Verification items for the finished model (mm, model axes). Face numbers are marked on the shaded views. Give positions to 0.01 mm unless a question says otherwise; leave off trailing zeros. Order: outer loops, then holes, each group sorted by start corner. A loop starts at its lowest first (then second) coordinate and runs counter-clockwise, first axis right, second up. Notation, with made-up numbers: (43, 72.5) - (51, 72.5) arc R24 ccw to (51, 106.5) - close; hole circle Ø5 at (-12, -5.75). An arc over 180 degrees is marked (long way). Answer as a JSON object with one key per item and string values. Group by question number.
(1) Section check B-B (x = -9.5). Record the boundary of the cut face in (y, z), then the cut area to 3 significant figures.
(2) Mould release check, pull along Z, two halves, no side actions. Record for the marked faces 1 and 2: +Z half, -Z half, draft (parallel to the pull), parting line (faces both ways), or undercut.
(3) Thickness scan on line 1 (X direction, y = 0.25, z = -8); line 2 (Z direction, x = -30, y = 1.65); line 3 (X direction, y = 2.35, z = -24). Record the ranges inside material, lowest first.
(4) Depth check by flat-ended pin: pin 1 Ø3.5 at (x, z) = (31.46, 22.98) entering from +Y; pin 2 Ø1.5 at (y, z) = (1, -19) entering from +X; pin 3 Ø1.7 at (y, z) = (1.5, -22) entering from +X; pin 4 Ø0.6 at (x, y) = (-1, 1) entering from +Z. Enter the tip coordinate at first touch or a pass-through.
(5) Section check A-A (z = 6.5). Record the boundary of the cut face in (x, y).
(6) Section check D-D (y = 3.45). Count the separate pieces of the cut face and the enclosed holes in it, then the cut area to 3 significant figures.
(7) Section check C-C (x = 31). Record the boundary of the cut face in (y, z), then the cut area to 3 significant figures.
```python
from build123d import *

# Parameters (mm, degrees)
SKETCH1_R           = 1.6
BOSS_EXTRUDE1_DEPTH = 4.1
CUT_EXTRUDE1_DEPTH  = 2
FILLET2_R           = 30
CUT_EXTRUDE4_DEPTH  = 3.1
SKETCH7_W           = 35
SKETCH7_H           = 20
CUT_EXTRUDE5_DEPTH  = 3.1


with BuildPart() as part:
    # Sketch1 → Boss-Extrude1 (new body)
    with BuildSketch(Plane(origin=(0, 0, 0), x_dir=(1, 0, 0), z_dir=(0, 1, 0))):
        Polygon((-12.5, 35), (12.5, 35), (23.684823703, 36.412745764), (36.412745764, 23.684823703), (35, 12.5), (35, -12.5), (36.412745764, -23.684823703), (23.684823703, -36.412745764), (12.5, -35), (-12.5, -35), (-23.684823703, -36.412745764), (-36.412745764, -23.684823703), (-35, -12.5), (-35, 12.5), (-36.412745764, 23.684823703), (-23.684823703, 36.412745764), align=None)
        with Locations((22.977716922, 31.462998296)):
            Circle(SKETCH1_R, mode=Mode.SUBTRACT)
        with Locations((31.462998296, 22.977716922)):
            Circle(SKETCH1_R, mode=Mode.SUBTRACT)
        with Locations((31.462998296, -22.977716922)):
            Circle(SKETCH1_R, mode=Mode.SUBTRACT)
        with Locations((22.977716922, -31.462998296)):
            Circle(SKETCH1_R, mode=Mode.SUBTRACT)
        with Locations((-22.977716922, -31.462998296)):
            Circle(SKETCH1_R, mode=Mode.SUBTRACT)
        with Locations((-31.462998296, -22.977716922)):
            Circle(SKETCH1_R, mode=Mode.SUBTRACT)
        with Locations((-31.462998296, 22.977716922)):
            Circle(SKETCH1_R, mode=Mode.SUBTRACT)
        with Locations((-22.977716922, 31.462998296)):
            Circle(SKETCH1_R, mode=Mode.SUBTRACT)
    extrude(amount=BOSS_EXTRUDE1_DEPTH)

    # Sketch2 → Cut-Extrude1 (cut)
    with BuildSketch(Plane(origin=(0, 4.1, 0), x_dir=(1, 0, 0), z_dir=(0, 1, 0))):
        Polygon((0, 0), (0, 29), (-4.760594582, 29), (-18.369647406, 29), (-29, 18.369647406), (-29, 0), align=None)
        Polygon((18.369647406, 29), (0, 29), (0, 0), (-29, 0), (-29, -18.369647406), (-18.369647406, -29), (18.369647406, -29), (29, -18.369647406), (29, 18.369647406), align=None)
    extrude(amount=-CUT_EXTRUDE1_DEPTH, mode=Mode.SUBTRACT)

    # Fillet2
    fillet2_edges = [part.edges().sort_by_distance(p)[0] for p in [
        (-12.5, 2.05, -35),
        (12.5, 2.05, -35),
        (35, 2.05, -12.5),
        (35, 2.05, 12.5),
        (12.5, 2.05, 35),
        (-12.5, 2.05, 35),
        (-35, 2.05, 12.5),
        (-35, 2.05, -12.5),
    ]]
    fillet(fillet2_edges, radius=FILLET2_R)

    # Sketch6 → Cut-Extrude4 (cut, through all)
    with BuildSketch(Plane(origin=(0, 2.1, 0), x_dir=(1, 0, 0), z_dir=(0, 1, 0))):
        with BuildLine():
            Line((-1.5, 19.7), (-1.5, 18.3))
            ThreePointArc((-1.5, 18.3), (-1.734314575, 17.734314575), (-2.3, 17.5))
            Line((-2.3, 17.5), (-6.7, 17.5))
            ThreePointArc((-6.7, 17.5), (-7.265685425, 17.734314575), (-7.5, 18.3))
            Line((-7.5, 18.3), (-7.5, 26.7))
            ThreePointArc((-7.5, 26.7), (-7.265685425, 27.265685425), (-6.7, 27.5))
            Line((-6.7, 27.5), (6.7, 27.5))
            ThreePointArc((6.7, 27.5), (7.265685425, 27.265685425), (7.5, 26.7))
            Line((7.5, 26.7), (7.5, 18.3))
            ThreePointArc((7.5, 18.3), (7.265685425, 17.734314575), (6.7, 17.5))
            Line((6.7, 17.5), (2.3, 17.5))
            ThreePointArc((2.3, 17.5), (1.734314575, 17.734314575), (1.5, 18.3))
            Line((1.5, 18.3), (1.5, 19.7))
            ThreePointArc((1.5, 19.7), (1.734314575, 20.265685425), (2.3, 20.5))
            Line((2.3, 20.5), (4.2, 20.5))
            ThreePointArc((4.2, 20.5), (4.765685425, 20.734314575), (5, 21.3))
            Line((5, 21.3), (5, 23.7))
            ThreePointArc((5, 23.7), (4.765685425, 24.265685425), (4.2, 24.5))
            Line((4.2, 24.5), (-4.2, 24.5))
            ThreePointArc((-4.2, 24.5), (-4.765685425, 24.265685425), (-5, 23.7))
            Line((-5, 23.7), (-5, 21.3))
            ThreePointArc((-5, 21.3), (-4.765685425, 20.734314575), (-4.2, 20.5))
            Line((-4.2, 20.5), (-2.3, 20.5))
            ThreePointArc((-2.3, 20.5), (-1.734314575, 20.265685425), (-1.5, 19.7))
        make_face()
        with BuildLine():
            Line((-1.5, -19.7), (-1.5, -18.3))
            ThreePointArc((-1.5, -18.3), (-1.734314575, -17.734314575), (-2.3, -17.5))
            Line((-2.3, -17.5), (-6.7, -17.5))
            ThreePointArc((-6.7, -17.5), (-7.265685425, -17.734314575), (-7.5, -18.3))
            Line((-7.5, -18.3), (-7.5, -26.7))
            ThreePointArc((-7.5, -26.7), (-7.265685425, -27.265685425), (-6.7, -27.5))
            Line((-6.7, -27.5), (6.7, -27.5))
            ThreePointArc((6.7, -27.5), (7.265685425, -27.265685425), (7.5, -26.7))
            Line((7.5, -26.7), (7.5, -18.3))
            ThreePointArc((7.5, -18.3), (7.265685425, -17.734314575), (6.7, -17.5))
            Line((6.7, -17.5), (2.3, -17.5))
            ThreePointArc((2.3, -17.5), (1.734314575, -17.734314575), (1.5, -18.3))
            Line((1.5, -18.3), (1.5, -19.7))
            ThreePointArc((1.5, -19.7), (1.734314575, -20.265685425), (2.3, -20.5))
            Line((2.3, -20.5), (4.2, -20.5))
            ThreePointArc((4.2, -20.5), (4.765685425, -20.734314575), (5, -21.3))
            Line((5, -21.3), (5, -23.7))
            ThreePointArc((5, -23.7), (4.765685425, -24.265685425), (4.2, -24.5))
            Line((4.2, -24.5), (-4.2, -24.5))
            ThreePointArc((-4.2, -24.5), (-4.765685425, -24.265685425), (-5, -23.7))
            Line((-5, -23.7), (-5, -21.3))
            ThreePointArc((-5, -21.3), (-4.765685425, -20.734314575), (-4.2, -20.5))
            Line((-4.2, -20.5), (-2.3, -20.5))
            ThreePointArc((-2.3, -20.5), (-1.734314575, -20.265685425), (-1.5, -19.7))
        make_face()
    extrude(amount=-CUT_EXTRUDE4_DEPTH, mode=Mode.SUBTRACT)

    # Sketch7 → Cut-Extrude5 (cut, through all)
    with BuildSketch(Plane(origin=(0, 2.1, 0), x_dir=(1, 0, 0), z_dir=(0, 1, 0))):
        Rectangle(SKETCH7_W, SKETCH7_H)
    extrude(amount=-CUT_EXTRUDE5_DEPTH, mode=Mode.SUBTRACT)


solid = part.part
```
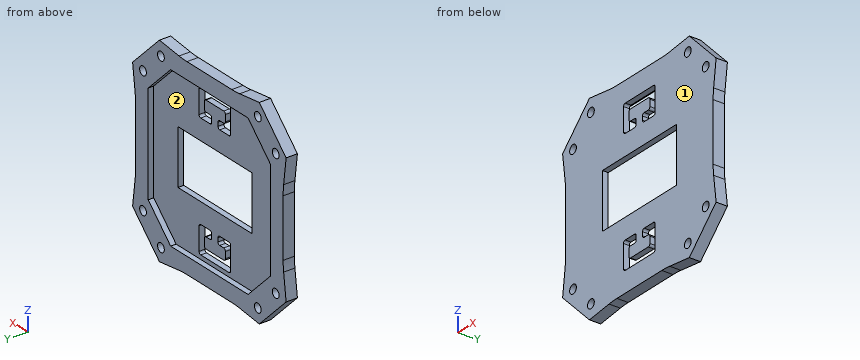
Solutions:
{
 "1": {"outline": "(0, -35) - (4.1, -35) - (4.1, -29) - (2.1, -29) - (2.1, -10) - (0, -10) - close; (0, 10) - (2.1, 10) - (2.1, 29) - (4.1, 29) - (4.1, 35) - (0, 35) - close", "area": "129 mm2"},
 "2": {"face 1": "draft", "face 2": "undercut"},
 "3": {"line 1": "x = -35 to -17.5, 17.5 to 35", "line 2": "z = -30.1 to -23.63, -22.33 to 22.33, 23.63 to 30.1", "line 3": "x = -36.1 to -32.69, -30.23 to -23.37, 23.37 to 30.23, 32.69 to 36.1"},
 "4": {"pin 1": "stops at y = 4.1", "pin 2": "stops at x = 35.92", "pin 3": "stops at x = 36.31", "pin 4": "stops at z = 35"},
 "5": {"outline": "(-35, 0) - (-17.5, 0) - (-17.5, 2.1) - (-29, 2.1) - (-29, 4.1) - (-35, 4.1) - close; (17.5, 0) - (35, 0) - (35, 4.1) - (29, 4.1) - (29, 2.1) - (17.5, 2.1) - close"},
 "6": {"separate pieces": "1", "enclosed holes": "9", "area": "1,570 mm2"},
 "7": {"outline": "(0, -29.1) - (4.1, -29.1) - (4.1, -24.51) - (0, -24.51) - close; (0, -21.45) - (4.1, -21.45) - (4.1, 21.45) - (0, 21.45) - close; (0, 24.51) - (4.1, 24.51) - (4.1, 29.1) - (0, 29.1) - close", "area": "213 mm2"}
}
